Check sheet for the modelled part. Datum: model origin and axes. Units: mm. A direction names the side the tool comes from. Give positions to 0.01 mm unless a question says otherwise; leave off trailing zeros. Write each loop counter-clockwise with the first axis right and the second up, starting at its lowest first coordinate (ties: lowest second). Pieces come first, ordered by that corner, then holes. Notation, with made-up numbers: M -40,45.25 L 14,45.25 A17 cw 14,69.25 Z; hole C 82,82.25 d9. An arc over 180 degrees is marked long. Use CSV: the item, a comma, the result in double quotes. Start each with the question number.
1. Depth check by flat-ended pin: P1, Ø4.5, axis at y = -34, z = -3, coming from the +X side; P2, Ø3, axis at y = -25.5, z = 17.5, coming from the +X side; P3, Ø22.5, axis at y = -35, z = 20.5, coming from the -X side. Enter the tip coordinate at first touch or a pass-through.
2. Scan lines: line 1 (Y direction, x = 13.5, z = 15.5); line 2 (Y direction, x = -12.75, z = 0); line 3 (X direction, y = -9, z = 20). Record each from-to range of solid material in increasing order.
3. Cross-section at A-A, the plane x = -50.5. Enter the section's corners in (y, z), and give its area (3 significant figures).
4. Cross-section at B-B, the plane x = 33. Enter the section's corners in (y, z), and give its area (3 significant figures).
5. Mould release check, pull along Y, two halves, no side actions. Record for faces 3 (the face through (49.86, 6.804, 1.511)), 4 (the face through (10.46, -34.8, -11.47)), 5 (the face through (10.465, -27.336, 24.404)): +Y half, -Y half, draft (parallel to the pull), parting line (faces both ways), or undercut.
6. Access from +Z, -Z, +X, -X, +Y, -Y to the whole of each face (thin tool, end or side, straight path). Record for faces 1 (the face through (-10.465, -26.98, -24.453)), 2 (the face through (8, -17, -33)).
from build123d import *

# Parameters (mm, degrees)
BOSS_EXTRUDE2_DEPTH  = 5
CIRPATTERN1_COUNT    = 6
MIRROR1_COPY_1_DEPTH = 5
MIRROR1_COPY_2_DEPTH = 5
MIRROR1_COPY_3_DEPTH = 5
MIRROR1_COPY_4_DEPTH = 5
MIRROR1_COPY_5_DEPTH = 5


with BuildPart() as part:
    # Sketch2 → Revolve1 (revolve)
    with BuildSketch(Plane.XY, mode=Mode.PRIVATE) as revolve1_sk:
        with BuildLine():
            Line((-22, 61.489125293), (-14, 50))
            Line((-14, 50), (-8, 50))
            ThreePointArc((-8, 50), (-5.656854249, 44.343145751), (0, 42))
            ThreePointArc((0, 42), (5.656854249, 44.343145751), (8, 50))
            Line((8, 50), (14, 50))
            Line((14, 50), (22, 61.489125293))
            ThreePointArc((22, 61.489125293), (0, 83.489125293), (-22, 61.489125293))
        make_face()
    revolve(revolve1_sk.sketch.rotate(Axis((0, 0, 0), (1, 0, 0)), 90), axis=Axis((0, 0, 0), (1, 0, 0)))

    # Sketch3 → Revolve2 (revolve)
    with BuildSketch(Plane.XY, mode=Mode.PRIVATE) as revolve2_sk:
        with BuildLine():
            Line((-27, 9.055449855), (-40, 9.055449855))
            Line((-40, 9.055449855), (-40, 6.969952313))
            Line((-40, 6.969952313), (-60, 6.969952313))
            Line((-60, 6.969952313), (-60, 0))
            Line((-60, 0), (60, 0))
            Line((60, 0), (60, 6.969952313))
            Line((60, 6.969952313), (40, 6.969952313))
            Line((40, 6.969952313), (40, 9.055449855))
            Line((40, 9.055449855), (27, 9.055449855))
            Line((27, 9.055449855), (27, 25))
            Line((27, 25), (15.652221366, 29.861325966))
            Line((15.652221366, 29.861325966), (8, 29.861325966))
            Line((8, 29.861325966), (8, 43.630803847))
            Line((8, 43.630803847), (16.135165196, 43.630803847))
            Line((16.135165196, 43.630803847), (16.135165196, 50))
            Line((16.135165196, 50), (8, 50))
            ThreePointArc((8, 50), (0, 42), (-8, 50))
            Line((-8, 50), (-16.135165196, 50))
            Line((-16.135165196, 50), (-16.135165196, 43.630803847))
            Line((-16.135165196, 43.630803847), (-8, 43.630803847))
            Line((-8, 43.630803847), (-8, 29.861325966))
            Line((-8, 29.861325966), (-15.652221366, 29.861325966))
            Line((-15.652221366, 29.861325966), (-27, 25))
            Line((-27, 25), (-27, 9.055449855))
        make_face()
    revolve(revolve2_sk.sketch.rotate(Axis((-27, 0, 0), (-1, 0, 0)), 90), axis=Axis((-27, 0, 0), (-1, 0, 0)))

    # Sketch4 → Boss-Extrude2 (add)
    with BuildSketch(Plane(origin=(8, 0, 0), x_dir=(0, 0, -1), z_dir=(1, 0, 0))):
        with BuildLine():
            Line((-49.891400962, 3.293646928), (-28.226766869, 9.744148017))
            ThreePointArc((-28.226766869, 9.744148017), (-29.860364168, -0.239666883), (-28.066722375, -10.19597389))
            Line((-28.066722375, -10.19597389), (-49.91509062, -2.912684053))
            ThreePointArc((-49.91509062, -2.912684053), (-49.999635764, 0.190849359), (-49.891400962, 3.293646928))
        make_face()
    boss_extrude2 = extrude(amount=BOSS_EXTRUDE2_DEPTH)

    # CirPattern1: Boss-Extrude2 ×6 about axis
    cirpattern1_axis = Axis((0, 0, 0), (1, 0, 0))
    for i in range(1, CIRPATTERN1_COUNT):
        add(boss_extrude2.rotate(cirpattern1_axis, i * 360 / CIRPATTERN1_COUNT))

    # Mirror1: Boss-Extrude2 across plane
    add(boss_extrude2.mirror(Plane(origin=(0, 0, 0), x_dir=(0, 0, 1), z_dir=(1, 0, 0))))

    # Mirror1 copy 1 sketch → Mirror1 copy 1 (add)
    with BuildSketch(Plane(origin=(-8, 0, 0), x_dir=(0, 0.8660254037844386, -0.5000000000000001), z_dir=(-1, 0, 0))):
        with BuildLine():
            Line((-49.891400962, -3.293646928), (-28.226766869, -9.744148017))
            ThreePointArc((-28.226766869, -9.744148017), (-29.860364168, 0.239666883), (-28.066722375, 10.19597389))
            Line((-28.066722375, 10.19597389), (-49.91509062, 2.912684053))
            ThreePointArc((-49.91509062, 2.912684053), (-49.999635764, -0.190849359), (-49.891400962, -3.293646928))
        make_face()
    extrude(amount=MIRROR1_COPY_1_DEPTH)

    # Mirror1 copy 2 sketch → Mirror1 copy 2 (add)
    with BuildSketch(Plane(origin=(-8, 0, 0), x_dir=(0, 0.8660254037844387, 0.4999999999999998), z_dir=(-1, 0, 0))):
        with BuildLine():
            Line((-49.891400962, -3.293646928), (-28.226766869, -9.744148017))
            ThreePointArc((-28.226766869, -9.744148017), (-29.860364168, 0.239666883), (-28.066722375, 10.19597389))
            Line((-28.066722375, 10.19597389), (-49.91509062, 2.912684053))
            ThreePointArc((-49.91509062, 2.912684053), (-49.999635764, -0.190849359), (-49.891400962, -3.293646928))
        make_face()
    extrude(amount=MIRROR1_COPY_2_DEPTH)

    # Mirror1 copy 3 sketch → Mirror1 copy 3 (add)
    with BuildSketch(Plane.ZY.offset(8)):
        with BuildLine():
            Line((-49.891400962, -3.293646928), (-28.226766869, -9.744148017))
            ThreePointArc((-28.226766869, -9.744148017), (-29.860364168, 0.239666883), (-28.066722375, 10.19597389))
            Line((-28.066722375, 10.19597389), (-49.91509062, 2.912684053))
            ThreePointArc((-49.91509062, 2.912684053), (-49.999635764, -0.190849359), (-49.891400962, -3.293646928))
        make_face()
    extrude(amount=MIRROR1_COPY_3_DEPTH)

    # Mirror1 copy 4 sketch → Mirror1 copy 4 (add)
    with BuildSketch(Plane(origin=(-8, 0, 0), x_dir=(0, -0.8660254037844384, 0.5000000000000004), z_dir=(-1, 0, 0))):
        with BuildLine():
            Line((-49.891400962, -3.293646928), (-28.226766869, -9.744148017))
            ThreePointArc((-28.226766869, -9.744148017), (-29.860364168, 0.239666883), (-28.066722375, 10.19597389))
            Line((-28.066722375, 10.19597389), (-49.91509062, 2.912684053))
            ThreePointArc((-49.91509062, 2.912684053), (-49.999635764, -0.190849359), (-49.891400962, -3.293646928))
        make_face()
    extrude(amount=MIRROR1_COPY_4_DEPTH)

    # Mirror1 copy 5 sketch → Mirror1 copy 5 (add)
    with BuildSketch(Plane(origin=(-8, 0, 0), x_dir=(0, -0.8660254037844386, -0.5000000000000001), z_dir=(-1, 0, 0))):
        with BuildLine():
            Line((-49.891400962, -3.293646928), (-28.226766869, -9.744148017))
            ThreePointArc((-28.226766869, -9.744148017), (-29.860364168, 0.239666883), (-28.066722375, 10.19597389))
            Line((-28.066722375, 10.19597389), (-49.91509062, 2.912684053))
            ThreePointArc((-49.91509062, 2.912684053), (-49.999635764, -0.190849359), (-49.891400962, -3.293646928))
        make_face()
    extrude(amount=MIRROR1_COPY_5_DEPTH)


solid = part.part
Worked answers:
1,P1,"stops at x = 8"
1,P2,"stops at x = 16.67"
1,P3,"stops at x = -16.94"
2,line 1,"y = -77.32 to -40.78, -25.52 to 25.52, 40.78 to 77.32"
2,line 2,"y = -79.42 to -43.63, -29.86 to 29.86, 43.63 to 79.42"
2,line 3,"x = -27 to 27"
3,outline,"C 0,0 d13.94"
3,area,"153 mm^2"
4,outline,"C 0,0 d18.11"
4,area,"258 mm^2"
5,face 3,"parting line"
5,face 4,"undercut"
5,face 5,"undercut"
6,face 1,"-X"
6,face 2,"+X"
